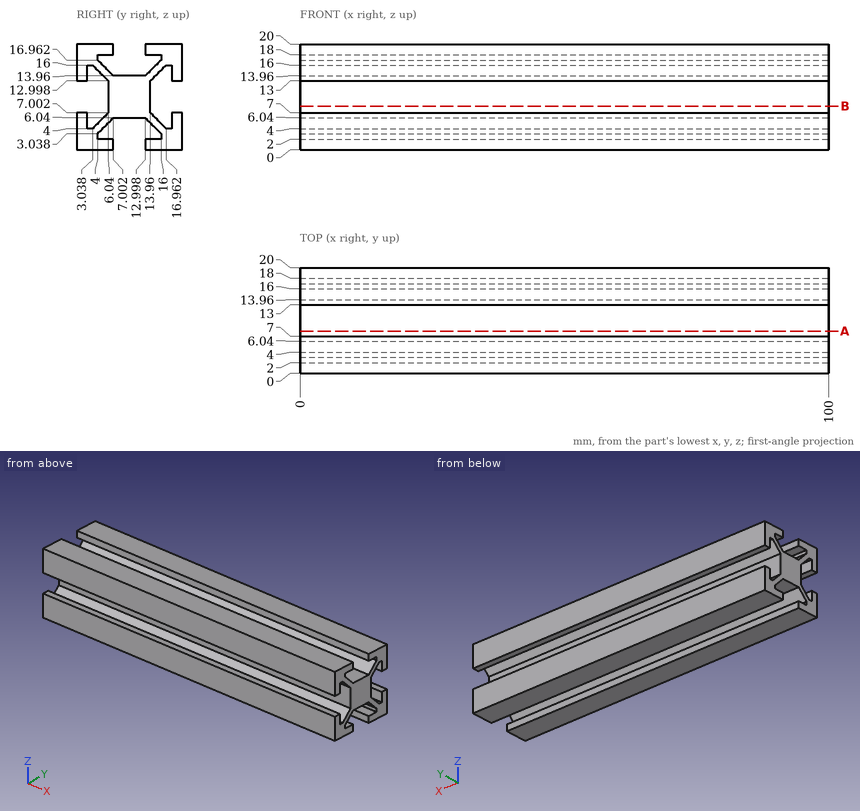
Here's the drawing with two shaded views (mm, measured from the low corner). I have some questions. Give positions to 0.01 mm unless a question says otherwise; leave off trailing zeros. Write each loop counter-clockwise with the first axis right and the second up, starting at its lowest first coordinate (ties: lowest second). Pieces come first, ordered by that corner, then holes. Notation, with made-up numbers: (-5, 57) -> (32, 57) arc R19 cw to (32, 79) -> close; hole circle Ø5 at (-38, -2). An arc over 180 degrees is marked (long way). Answer as a JSON object with one key per item and string values. Group by question number.
Item 1: Suppose I cut it at A-A (y = 8). Please give me the cut outline in (x, z), plus the area to 3 significant figures.
Item 2: I'm going to push a flat-ended pin straight in: P1, Ø4, axis at x = 28.5, z = 10, coming from the -Y side. Where does the tip first touch, or does it pass through?
Item 3: Please list where these lines run through material, in increasing order: line 1 (Z direction, x = 15, y = 19); line 2 (Z direction, x = 63, y = 2.75); line 3 (Z direction, x = 53, y = 13.25). Write a range as [from, to].
Findings:
{
 "1": {"outline": "(0, 6.04) -> (100, 6.04) -> (100, 13.96) -> (0, 13.96) -> close", "area": "792 mm²"},
 "2": {"P1": "stops at y = 6.04"},
 "3": {"line 1": "z = [0, 7], [13, 20]", "line 2": "z = [0, 4], [16, 20]", "line 3": "z = [0, 2], [5.79, 14.21], [18, 20]"}
}
